from build123d import *

# Parameters (mm, degrees)
SKETCH1_R           = 1
BOSS_EXTRUDE1_DEPTH = 2.5
SKETCH2_R           = 5.5
SKETCH2_R_2         = 3
BOSS_EXTRUDE3_DEPTH = 4.25
CUT_EXTRUDE1_REACH  = 4.5
SKETCH4_R           = 3
CHAMFER1_SIZE       = 1


with BuildPart() as part:
    # Sketch1 → Boss-Extrude1 (new body)
    with BuildSketch(Plane(origin=(0, 0, 0), x_dir=(1, 0, 0), z_dir=(0, 1, 0))):
        with BuildLine():
            ThreePointArc((6.5, 0), (0, 6.5), (-6.5, 0))
            Line((-6.5, 0), (-6.457689178, -0.740439382))
            Line((-6.457689178, -0.740439382), (-5.5, -17.5))
            Line((-5.5, -17.5), (5.5, -17.5))
            Line((5.5, -17.5), (6.457689178, -0.740439382))
            Line((6.457689178, -0.740439382), (6.5, 0))
        make_face()
        with Locations((0, -16)):
            Circle(SKETCH1_R, mode=Mode.SUBTRACT)
        with Locations((0, -10)):
            Circle(SKETCH1_R, mode=Mode.SUBTRACT)
    extrude(amount=BOSS_EXTRUDE1_DEPTH)

    # Sketch2 → Boss-Extrude3 (add)
    with BuildSketch(Plane(origin=(0, 2.5, 0), x_dir=(1, 0, 0), z_dir=(0, 1, 0))):
        Circle(SKETCH2_R)
        Circle(SKETCH2_R_2, mode=Mode.SUBTRACT)
    extrude(amount=BOSS_EXTRUDE3_DEPTH)

    # Sketch4 → Cut-Extrude1 (cut, up to next)
    with BuildSketch(Plane(origin=(0, 2.5, 0), x_dir=(1, 0, 0), z_dir=(0, 1, 0)), mode=Mode.PRIVATE) as cut_extrude1_sk1:
        Circle(SKETCH4_R)
    cut_extrude1_tool1 = extrude(cut_extrude1_sk1.sketch, amount=-CUT_EXTRUDE1_REACH, mode=Mode.PRIVATE) & part.part
    add(cut_extrude1_tool1.solids().sort_by_distance((0, 2.5, 0))[0], mode=Mode.SUBTRACT)

    # Chamfer1
    chamfer1_edges = [part.edges().sort_by_distance(p)[0] for p in [
        (-5.5, 6.75, 0),
    ]]
    chamfer(chamfer1_edges, length=CHAMFER1_SIZE)


solid = part.part
Read the model definition and answer for the solid it produces. Units are mm, in the model's axes. Round coordinates to 2 decimals unless told otherwise and drop trailing zeros. Loops run counter-clockwise (first coordinate to the right, second up) from the corner with the lowest first, then second, coordinate; pieces in that order, holes last.
Q1. Section A-A on x = 0 is taken. Write down the section's boundary in (y, z).
Q2. Section B-B on y = 1.25 is taken. Write down the section's boundary in (x, z), and give its area (3 significant figures).
Q3. Each of these flat-tipped pins is pushed along its axis until it touches: pin 1 (2 mm diameter, centred on y = 4, z = 10.5, fed in from +X); pin 2 (4 mm diameter, centred on x = -5, z = 5.5, fed in from -Y); pin 3 (2 mm diameter, centred on x = -4.5, y = 4, fed in from -Z); pin 4 (2.5 mm diameter, centred on x = 0, z = 10, fed in from +Y). Where does it stop, or does it pass through?
Q4. Consider probe 1 along Z at (x, y) = (0, 1.9); probe 2 along X at (y, z) = (3.9, 0). Determine where each line is inside the solid, lowest interval first.
Q5. Section D-D on y = 6.25 is taken. Write down the section's boundary in (x, z), and give its area (3 significant figures).
Q6. Determine the mould class of faces 1 (the face through (0, 2.5, 8)), 2 (the face through (-1.19, 4.1, 5.37)), 3 (the face through (0, 1, 9)) for opening direction Z: released by +Z, released by -Z, zero draft, split by the parting line, or undercut.
Q7. Section C-C on z = 10 is taken. Write down the section's boundary in (x, y), and give its area (3 significant figures).
Output:
1. outline: (0, -6.5) - (2.5, -6.5) - (2.5, -5.5) - (5.75, -5.5) - (6.75, -4.5) - (6.75, -3) - (0, -3) - close; (0, 3) - (6.75, 3) - (6.75, 4.5) - (5.75, 5.5) - (2.5, 5.5) - (2.5, 9) - (0, 9) - close; (0, 11) - (2.5, 11) - (2.5, 15) - (0, 15) - close; (0, 17) - (2.5, 17) - (2.5, 17.5) - (0, 17.5) - close
2. outline: (-6.5, 0) arc R6.5 ccw to (6.5, 0) - (5.5, 17.5) - (-5.5, 17.5) - close; hole circle Ø6 at (0, 0); hole circle Ø2 at (0, 10); hole circle Ø2 at (0, 16)
2. area: 242 mm2
3. pin 1: passes through
3. pin 2: stops at y = 0
3. pin 3: stops at z = -4.24
3. pin 4: stops at y = 2.5
4. probe 1: z = -6.5 to -3, 3 to 9, 11 to 15, 17 to 17.5
4. probe 2: x = -5.5 to -3, 3 to 5.5
5. outline: circle Ø10 at (0, 0); hole circle Ø6 at (0, 0)
5. area: 50.3 mm2
6. face 1: zero draft
6. face 2: split by the parting line
6. face 3: undercut
7. outline: (-5.93, 0) - (-1, 0) - (-1, 2.5) - (-5.93, 2.5) - close; (1, 0) - (5.93, 0) - (5.93, 2.5) - (1, 2.5) - close
7. area: 24.6 mm2
